Study the drawing (mm; zero at the part's minimum x, y, z) and answer. A direction names the side the tool comes from. Round coordinates to 2 decimals unless told otherwise and drop trailing zeros. Write each loop counter-clockwise with the first axis right and the second up, starting at its lowest first coordinate (ties: lowest second). Pieces come first, ordered by that corner, then holes. Notation, with made-up numbers: (-13.5, -8) -> (32.5, -8) arc R27 cw to (32.5, 10) -> close; hole circle Ø11 at (81.25, 48.25). An arc over 180 degrees is marked (long way). Return JSON: item names as keys, results as strings.
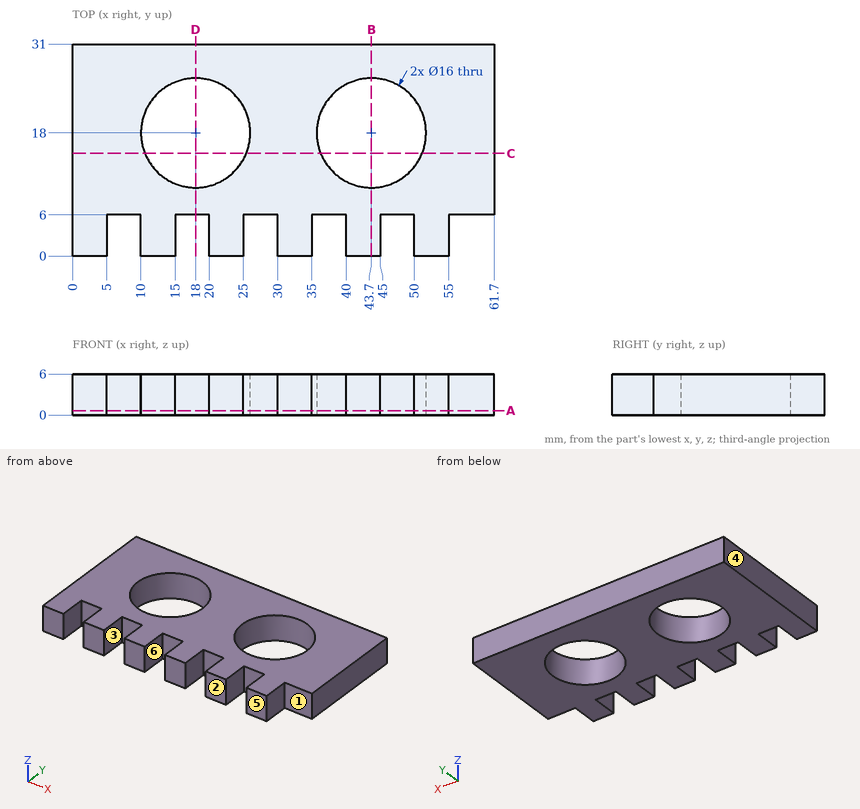
Item 1: Section D-D (x = 18) is taken. Give the vertices of the cut face in (y, z), then the cut area to 3 significant figures.
Worked answers:
{"outline": "(6, 0) -> (10, 0) -> (10, 6) -> (6, 6) -> close; (26, 0) -> (31, 0) -> (31, 6) -> (26, 6) -> close", "area": "54.0 mm2"}
Item 2: Straight lines are drawn through the part: L1, parallel to X at y = 3, z = 1.25; L2, parallel to Y at x = 43.7, z = 1.5; L3, parallel to Y at x = 18, z = 2.6. For each, find the intervals that lie inside material, in ascending order. Write a range as [from, to].
Worked answers:
{"L1": "x = [0, 5], [10, 15], [20, 25], [30, 35], [40, 45], [50, 55]", "L2": "y = [0, 10], [26, 31]", "L3": "y = [6, 10], [26, 31]"}
Item 3: A tool of negligible diameter and unlimited length cuts with its end or side. For the marked faces 1, 2 and 3, from which of +Z, -Z, +X, -X, +Y, -Y can it reach the whole face along a straight path? Write none if from no direction.
Worked answers:
{"face 1": "+Z, -Z, +X, -Y", "face 2": "+Z, -Z, +X, -X, -Y", "face 3": "+Z, -Z, -Y"}
Item 4: For a pull along X with two mould halves and no side action, classify the marked faces 4, 5 and 6 as released by +X, released by -X, zero draft, split by the parting line, or undercut.
Worked answers:
{"face 4": "released by -X", "face 5": "zero draft", "face 6": "undercut"}
Item 5: Section B-B (x = 43.7) is taken. Give the vertices of the cut face in (y, z), then the cut area to 3 significant figures.
Worked answers:
{"outline": "(0, 0) -> (10, 0) -> (10, 6) -> (0, 6) -> close; (26, 0) -> (31, 0) -> (31, 6) -> (26, 6) -> close", "area": "90.0 mm2"}
Item 6: Section C-C (y = 15) is taken. Give the vertices of the cut face in (x, z), then the cut area to 3 significant figures.
Worked answers:
{"outline": "(0, 0) -> (10.58, 0) -> (10.58, 6) -> (0, 6) -> close; (25.42, 0) -> (36.28, 0) -> (36.28, 6) -> (25.42, 6) -> close; (51.12, 0) -> (61.7, 0) -> (61.7, 6) -> (51.12, 6) -> close", "area": "192 mm2"}
Item 7: Flat-ended cylindrical pins translate along their axes: pin 1 (1.8 mm diameter, centred on y = 4, z = 1.5, fed in from +X); pin 2 (14.5 mm diameter, centred on x = 18, y = 18, fed in from +Z); pin 3 (2.5 mm diameter, centred on x = 8, z = 2, fed in from -Y). Find the tip coordinate at first contact, or state that the pin passes through.
Worked answers:
{"pin 1": "stops at x = 55", "pin 2": "passes through", "pin 3": "stops at y = 6"}
Item 8: Section A-A (z = 0.65) is taken. Give the vertices of the cut face in (x, y).
Worked answers:
{"outline": "(0, 0) -> (5, 0) -> (5, 6) -> (10, 6) -> (10, 0) -> (15, 0) -> (15, 6) -> (20, 6) -> (20, 0) -> (25, 0) -> (25, 6) -> (30, 6) -> (30, 0) -> (35, 0) -> (35, 6) -> (40, 6) -> (40, 0) -> (45, 0) -> (45, 6) -> (50, 6) -> (50, 0) -> (55, 0) -> (55, 6) -> (61.7, 6) -> (61.7, 31) -> (0, 31) -> close; hole circle Ø16 at (18, 18); hole circle Ø16 at (43.7, 18)"}
